The model under review builds one solid part; all positions refer to its coordinate system, in mm. A direction names the side the tool comes from. Coordinates: 2 decimals unless noted, no trailing zeros. Loops run counter-clockwise (first coordinate to the right, second up) from the corner with the lowest first, then second, coordinate; pieces in that order, holes last. Notation, with made-up numbers: M 84.25,84.25 L 134.25,84.25 A21 cw 134.25,97.25 Z; hole C 51.25,22.25 d9. An arc over 180 degrees is marked long. Return JSON: item names as keys, results as strings.
```python
from build123d import *

# Parameters (mm, degrees)
SKETCH1_R           = 3.75
BOSS_EXTRUDE1_DEPTH = 25
FILLET1_R           = 2
SKETCH2_R           = 5.25
BOSS_EXTRUDE2_DEPTH = 2
FILLET2_R           = 2


with BuildPart() as part:
    # Sketch1 → Boss-Extrude1 (new body)
    with BuildSketch(Plane(origin=(0, 0, 0), x_dir=(1, 0, 0), z_dir=(0, 1, 0))):
        with Locations(Location((0, 0, 0), (0, 0, 270))):
            Circle(SKETCH1_R)
    extrude(amount=BOSS_EXTRUDE1_DEPTH)

    # Fillet1
    fillet1_edges = [part.edges().sort_by_distance(p)[0] for p in [
        (0, 25, -3.75),
    ]]
    fillet(fillet1_edges, radius=FILLET1_R)

    # Sketch2 → Boss-Extrude2 (add)
    with BuildSketch(Plane.XZ):
        with Locations(Location((0, 0, 0), (0, 0, 270))):
            Circle(SKETCH2_R)
    extrude(amount=BOSS_EXTRUDE2_DEPTH)

    # Fillet2
    # the kernel refuses this fillet: 2 mm, written as the material it adds along each edge
    with BuildSketch(Plane(origin=(0, 0, 0), x_dir=(0, 0, 1), z_dir=(-1, 0, 0))) as fillet2_piece_1:
        with BuildLine():
            CenterArc((5.75, 1.936491673), FILLET2_R, 180, 75.522487814)
            Line((3.75, 1.936491673), (3.71, 1.936491673))
            Line((3.71, 1.936491673), (3.71, 0))
            Line((3.71, 0), (3.75, -0.04))
            ThreePointArc((3.75, -0.04), (4.5, -0.04), (5.24, -0.038729833))
            Line((5.24, -0.038729833), (5.25, 0))
        make_face()
    revolve(axis=Axis((0, 0, 0), (0, 1, 0)))


solid = part.part
```
1. Machinability: for faces 1 (the face through (1.6, -1, -5)), 2 (the face through (0.165, 12.321, -3.746)), which of the approach directions +Z, -Z, +X, -X, +Y, -Y give a long, thin tool a straight path to every point of the face, cutting with its end or side? Answer none if there is none.
Check values:
{"face 1": "+Y, -Y", "face 2": "+Y"}
2. To check wall thickness, follow line 1 (Y direction, x = 0.5, z = 4); line 2 (Z direction, x = -2.75, y = 5.25); line 3 (Y direction, x = 1.5, z = -3). State the ranges of each line that lie inside material, in increasing order.
Check values:
{"line 1": "-2 to 0.91", "line 2": "-2.55 to 2.55", "line 3": "-2 to 24.19"}
3. Add section A-A on y = 19. Give the boundary of the cut face in (x, z), plus the area to 3 significant figures.
Check values:
{"outline": "C 0,0 d7.5", "area": "44.2 mm²"}
4. Insertion check: pin 1 Ø6 at (x, y) = (1.5, 12) entering from -Z; pin 2 Ø3 at (y, z) = (19, 3.5) entering from -X; pin 3 Ø1.5 at (x, z) = (2.5, 2) entering from +Y. Each pin has a flat end and moves straight along its axis. Give the tip position at first contact, or say it passes through.
Check values:
{"pin 1": "z = -3.75", "pin 2": "x = -3.17", "pin 3": "y = 24.87"}
